```python
from build123d import *

# Parameters (mm, degrees)
SKETCH_3_R           = 9.5
CUT_EXTRUDE_1_DEPTH  = 321.526909947
SKETCH_4_R           = 9.5
CUT_EXTRUDE_2_DEPTH  = 321.526909947
SKETCH_5_R           = 9.5
CUT_EXTRUDE_3_DEPTH  = 321.526909947
SKETCH_6_R           = 9.5
CUT_EXTRUDE_4_DEPTH  = 321.526909947
SKETCH_7_R           = 9.5
CUT_EXTRUDE_5_DEPTH  = 321.526909947
SKETCH_8_R           = 9.5
CUT_EXTRUDE_6_DEPTH  = 321.526909947
SKETCH_9_R           = 9.5
CUT_EXTRUDE_7_DEPTH  = 321.526909947
SKETCH_10_R          = 9.5
CUT_EXTRUDE_8_DEPTH  = 321.526909947
SKETCH_11_R          = 9.5
CUT_EXTRUDE_9_DEPTH  = 321.526909947
SKETCH_12_R          = 9.5
CUT_EXTRUDE_10_DEPTH = 321.526909947
SKETCH_13_R          = 9.5
CUT_EXTRUDE_11_DEPTH = 321.526909947
SKETCH_14_R          = 9.5
CUT_EXTRUDE_12_DEPTH = 321.526909947


with BuildPart() as part:
    # Эскиз1 → Повернуть1 (revolve)
    with BuildSketch(Plane.XY, mode=Mode.PRIVATE) as revolve_1_sk:
        Polygon((0, 0), (265, 0), (265, 127.5), (239, 127.5), (239, 100), (239, 95), (220, 95), (220, 94), (200, 94), (144, 65.5), (70, 65.5), (25, 41), (1.5, 41), (3, 45), (0, 45), align=None)
    revolve(revolve_1_sk.sketch.rotate(Axis((0, 0, 0), (1, 0, 0)), 90), axis=Axis((0, 0, 0), (1, 0, 0)))

    # Эскиз2 → Вырез-Повернуть1 (revolve, cut)
    with BuildSketch(Plane.XY, mode=Mode.PRIVATE) as cut_revolve_1_sk:
        with BuildLine():
            Line((0, 0), (215.831336185, 0))
            Line((215.831336185, 0), (215.831336185, 52.583474267))
            Line((215.831336185, 52.583474267), (133.831336185, 52.583474267))
            Line((133.831336185, 52.583474267), (128.830273914, 52.583474267))
            ThreePointArc((128.830273914, 52.583474267), (122.304621517, 52.09322577), (115.89038393, 50.796291315))
            Line((115.89038393, 50.796291315), (42, 31))
            Line((42, 31), (0, 31))
            Line((0, 31), (0, 0))
        make_face()
    revolve(cut_revolve_1_sk.sketch.rotate(Axis((0, 0, 0), (1, 0, 0)), 90), axis=Axis((0, 0, 0), (1, 0, 0)), mode=Mode.SUBTRACT)

    # Эскиз3 → Вырез-Вытянуть1 (cut, through all)
    with BuildSketch(Plane(origin=(0, 0, 0), x_dir=(0, 0, -1), z_dir=(1, 0, 0))):
        with Locations((0, 113)):
            Circle(SKETCH_3_R)
    extrude(amount=CUT_EXTRUDE_1_DEPTH, mode=Mode.SUBTRACT)

    # Эскиз4 → Вырез-Вытянуть2 (cut, through all)
    with BuildSketch(Plane(origin=(0, 0, 0), x_dir=(0, 0, -1), z_dir=(1, 0, 0))):
        with Locations((-56.5, 97.860870628)):
            Circle(SKETCH_4_R)
    extrude(amount=CUT_EXTRUDE_2_DEPTH, mode=Mode.SUBTRACT)

    # Эскиз5 → Вырез-Вытянуть3 (cut, through all)
    with BuildSketch(Plane(origin=(0, 0, 0), x_dir=(0, 0, -1), z_dir=(1, 0, 0))):
        with Locations((-97.860870628, 56.5)):
            Circle(SKETCH_5_R)
    extrude(amount=CUT_EXTRUDE_3_DEPTH, mode=Mode.SUBTRACT)

    # Эскиз6 → Вырез-Вытянуть4 (cut, through all)
    with BuildSketch(Plane(origin=(0, 0, 0), x_dir=(0, 0, -1), z_dir=(1, 0, 0))):
        with Locations((-113, 0)):
            Circle(SKETCH_6_R)
    extrude(amount=CUT_EXTRUDE_4_DEPTH, mode=Mode.SUBTRACT)

    # Эскиз7 → Вырез-Вытянуть5 (cut, through all)
    with BuildSketch(Plane(origin=(0, 0, 0), x_dir=(0, 0, -1), z_dir=(1, 0, 0))):
        with Locations((-97.860870628, -56.5)):
            Circle(SKETCH_7_R)
    extrude(amount=CUT_EXTRUDE_5_DEPTH, mode=Mode.SUBTRACT)

    # Эскиз8 → Вырез-Вытянуть6 (cut, through all)
    with BuildSketch(Plane(origin=(0, 0, 0), x_dir=(0, 0, -1), z_dir=(1, 0, 0))):
        with Locations((-56.5, -97.860870628)):
            Circle(SKETCH_8_R)
    extrude(amount=CUT_EXTRUDE_6_DEPTH, mode=Mode.SUBTRACT)

    # Эскиз9 → Вырез-Вытянуть7 (cut, through all)
    with BuildSketch(Plane(origin=(0, 0, 0), x_dir=(0, 0, -1), z_dir=(1, 0, 0))):
        with Locations((0, -113)):
            Circle(SKETCH_9_R)
    extrude(amount=CUT_EXTRUDE_7_DEPTH, mode=Mode.SUBTRACT)

    # Эскиз10 → Вырез-Вытянуть8 (cut, through all)
    with BuildSketch(Plane(origin=(0, 0, 0), x_dir=(0, 0, -1), z_dir=(1, 0, 0))):
        with Locations((56.5, -97.860870628)):
            Circle(SKETCH_10_R)
    extrude(amount=CUT_EXTRUDE_8_DEPTH, mode=Mode.SUBTRACT)

    # Эскиз11 → Вырез-Вытянуть9 (cut, through all)
    with BuildSketch(Plane(origin=(0, 0, 0), x_dir=(0, 0, -1), z_dir=(1, 0, 0))):
        with Locations((97.860870628, -56.5)):
            Circle(SKETCH_11_R)
    extrude(amount=CUT_EXTRUDE_9_DEPTH, mode=Mode.SUBTRACT)

    # Эскиз12 → Вырез-Вытянуть10 (cut, through all)
    with BuildSketch(Plane(origin=(0, 0, 0), x_dir=(0, 0, -1), z_dir=(1, 0, 0))):
        with Locations((113, 0)):
            Circle(SKETCH_12_R)
    extrude(amount=CUT_EXTRUDE_10_DEPTH, mode=Mode.SUBTRACT)

    # Эскиз13 → Вырез-Вытянуть11 (cut, through all)
    with BuildSketch(Plane(origin=(0, 0, 0), x_dir=(0, 0, -1), z_dir=(1, 0, 0))):
        with Locations((97.860870628, 56.5)):
            Circle(SKETCH_13_R)
    extrude(amount=CUT_EXTRUDE_11_DEPTH, mode=Mode.SUBTRACT)

    # Эскиз14 → Вырез-Вытянуть12 (cut, through all)
    with BuildSketch(Plane(origin=(0, 0, 0), x_dir=(0, 0, -1), z_dir=(1, 0, 0))):
        with Locations((56.5, 97.860870628)):
            Circle(SKETCH_14_R)
    extrude(amount=CUT_EXTRUDE_12_DEPTH, mode=Mode.SUBTRACT)


solid = part.part
```
Source: CAD feature listing. Evaluate the final solid. Frame: model axes, mm. A direction names the side the tool comes from. Coordinates: 2 decimals unless noted, no trailing zeros. Loops run counter-clockwise (first coordinate to the right, second up) from the corner with the lowest first, then second, coordinate; pieces in that order, holes last. Notation, with made-up numbers: M -10.75,43 L -4.75,43 A5 ccw -4.75,48 Z; hole C 59.5,55.25 d2. An arc over 180 degrees is marked long. Use CSV: the item, a comma, the result in double quotes.
(1) Reachability of faces 1 (the face through (251.82, -62.28, 105.4)), 2 (the face through (239, -95, -10)), 3 (the face through (70.2, 34.2, 17.8)) from +Z, -Z, +X, -X, +Y, -Y: full face, straight path, thin tool, end or side. Return the list, or none.
Answers follow:
face 1,"+X, -X"
face 2,"-X"
face 3,"none"
(2) Line query: line 1 (Y direction, x = 246.5, z = 56.5); line 2 (X direction, y = 91, z = -80.5); line 3 (Z direction, x = 38, y = -21). Output: solid intervals per line, ascending. Write a range as [from, to].
Answers follow:
line 1,"[-114.3, -107.36], [-88.36, 88.36], [107.36, 114.3]"
line 2,"[239, 265]"
line 3,"[-43.25, -22.8], [22.8, 43.25]"
(3) Contact query for flat-ended pins moving along their axis: pin 1 (8 mm diameter, centred on y = 98, z = -88.5, fed in from +X); pin 2 (22 mm diameter, centred on y = 113, z = 0, fed in from +X); pin 3 (22 mm diameter, centred on y = -56.5, z = 97.86, fed in from -X); pin 4 (6 mm diameter, centred on x = 71.5, z = 3.5, fed in from +Y). Output: stop coordinate, or through.
Answers follow:
pin 1,"through"
pin 2,"x = 265"
pin 3,"x = 239"
pin 4,"y = 65.5"
(4) Cut plane A-A on y = -113. Return loops of the section in (x, z), and give its area (3 significant figures).
Answers follow:
outline,"M 239,-59.05 L 265,-59.05 L 265,-9.5 L 239,-9.5 Z; M 239,9.5 L 265,9.5 L 265,59.05 L 239,59.05 Z"
area,"2,580 mm²"
(5) Cut plane B-B on z = 0. Give the number of separate pieces and of enclosed holes in the cut face, and give its area (3 significant figures).
Answers follow:
separate pieces,"3"
enclosed holes,"0"
area,"19,400 mm²"
(6) Cut plane C-C on x = 205. Return loops of the section in (y, z), and give its area (3 significant figures).
Answers follow:
outline,"C 0,0 d188; hole C 0,0 d105.17"
area,"19,100 mm²"
(7) Draft query along X for faces 4 (the face through (215.831, -1, 1)), 5 (the face through (146.719, -20.09, 63.795)), 6 (the face through (209.86, -93.2, -12.24)). Return one class per face: pulls with the +X half, pulls with the -X half, needs draft (parallel to the pull), parting line crosses it, or undercut.
Answers follow:
face 4,"undercut"
face 5,"pulls with the -X half"
face 6,"needs draft"
